Geometry check sheet. Reference: the model listing, model coordinates, mm. Coordinates: 2 decimals unless noted, no trailing zeros. Order: outer loops, then holes, each group sorted by start corner. A loop starts at its lowest first (then second) coordinate and runs counter-clockwise, first axis right, second up. Notation, with made-up numbers: (87, -5) - (95, -5) arc R31 ccw to (95, 30) - close; hole circle Ø7 at (2, 65.5). An arc over 180 degrees is marked (long way). Put each result on its own line as item: value.
from build123d import *

# Parameters (mm, degrees)
SKETCH2_R                = 4
BOSS_EXTRUDE1_DEPTH      = 100
BOSS_EXTRUDE1_2_DEPTH    = 100
BOSS_EXTRUDE3_DEPTH      = 50
BOSS_EXTRUDE3_DEPTH_BACK = 175
BOSS_EXTRUDE4_START      = -15
SKETCH5_R                = 45.011707972
BOSS_EXTRUDE4_DEPTH      = 15
SKETCH8_R                = 30.011707972
CUT_EXTRUDE1_DEPTH       = 210


with BuildPart() as part:
    # Sketch2 → Boss-Extrude1 (new body)
    with BuildSketch(Plane(origin=(0, 0, 0), x_dir=(-1, 0, 0), z_dir=(0, 0.499999999999998, -0.8660254037844398))):
        with Locations(Location((-17.5, 0, 0), (0, 0, 90))):
            Circle(SKETCH2_R)
    boss_extrude1 = extrude(amount=BOSS_EXTRUDE1_DEPTH)



with BuildPart() as body_2:
    # Sketch2 → Boss-Extrude1 2 (new body)
    with BuildSketch(Plane(origin=(0, 0, 0), x_dir=(-1, 0, 0), z_dir=(0, 0.499999999999998, -0.8660254037844398))):
        with Locations(Location((17.5, 0, 0), (0, 0, 90))):
            Circle(SKETCH2_R)
    boss_extrude1_2 = extrude(amount=BOSS_EXTRUDE1_2_DEPTH)


with BuildPart() as part_1:
    add(part.part)

    add(body_2.part)  # Boss-Extrude3 merges body 2
    # Sketch4 → Boss-Extrude3 (add, two sides: drawn at the far end of the back side and taken through both)
    with BuildSketch(Plane(origin=(0, 0, 0), x_dir=(0, 0, 1), z_dir=(-0.9961946980917461, 0.08715574274765156, 0)).offset(-BOSS_EXTRUDE3_DEPTH_BACK)):
        with BuildLine():
            Line((80.028265546, 0), (65.028265546, 0))
            ThreePointArc((65.028265546, 0), (23.531574155, -27.727202731), (13.795075351, 21.221482222))
            Line((13.795075351, 21.221482222), (3.188473633, 31.82808394))
            ThreePointArc((3.188473633, 31.82808394), (17.79132267, -41.585395719), (80.028265546, 0))
        make_face()
    extrude(amount=BOSS_EXTRUDE3_DEPTH + BOSS_EXTRUDE3_DEPTH_BACK)

    # Sketch5 → Boss-Extrude4 (add)
    with BuildSketch(Plane(origin=(-49.809734905, 4.357787137, 0), x_dir=(0, 0, 1), z_dir=(-0.9961946980917462, 0.08715574274765156, 0)).offset(BOSS_EXTRUDE4_START)):
        with Locations(Location((35.016557573, 0, 0), (0, 0, 135))):
            Circle(SKETCH5_R)
    extrude(amount=BOSS_EXTRUDE4_DEPTH)

    # Mirror2: Boss-Extrude1, Boss-Extrude1 2 across plane
    add(boss_extrude1.mirror(Plane(origin=(0, 0, 35.016557573), x_dir=(1, 0, 0), z_dir=(0, 0, -1))))
    add(boss_extrude1_2.mirror(Plane(origin=(0, 0, 35.016557573), x_dir=(1, 0, 0), z_dir=(0, 0, -1))))

    # Sketch8 → Cut-Extrude1 (cut)
    with BuildSketch(Plane(origin=(174.334072166, -15.252254981, 0), x_dir=(0, 0, -1), z_dir=(0.9961946980917462, -0.08715574274765156, 0))):
        with Locations((-35.016557573, 0)):
            Circle(SKETCH8_R)
        with BuildLine():
            Line((-80.028265546, 0), (-208.366954173, 0))
            ThreePointArc((-208.366954173, 0), (87.560683384, -122.577240957), (-35.016557573, 173.3503966))
            Line((-35.016557573, 173.3503966), (-35.016557573, 45.011707972))
            ThreePointArc((-35.016557573, 45.011707972), (-3.188473633, -31.82808394), (-80.028265546, 0))
        make_face()
    extrude(amount=-CUT_EXTRUDE1_DEPTH, mode=Mode.SUBTRACT)


solid = part_1.part
Q1. Section check C-C on z = 47. Record the boundary of the cut face in (x, y).
Answer block:
outline: (-53.59, -38.86) - (170.55, -58.47) - (171.94, -42.66) - (-37.26, -24.36) - (-31.09, 46.27) - (-46.03, 47.58) - close
Q2. Draft check along Z on faces 1 (the cylindrical face through (68.755, -34.155, 24.298)), 2 (the flat face through (-17.444, 49.952, 156.664)), 3 (the flat face through (-49.755, 4.986, 34.386)), 4 (the flat face through (17.556, 0.781, 69.582)). Enter one of: pulls with the +Z half, pulls with the -Z half, needs draft (parallel to the pull), parting line crosses it, or undercut.
Answer block:
face 1: undercut
face 2: pulls with the +Z half
face 3: needs draft
face 4: undercut
Q3. Thickness scan on L1, parallel to Z at x = 67.5, y = -7; L2, parallel to Z at x = -36.5, y = -24; L3, parallel to X at y = -13.5, z = 20.5. Record the ranges inside material, lowest first. Write a range as [from, to].
Answer block:
L1: z = [-9.98, 5.02], [65.01, 80.02]
L2: z = [-0.93, 22.1], [47.93, 70.96]
L3: x = [-51.37, -36.31]
Q4. Section check A-A on z = 22.5. Record the boundary of the cut face in (x, y), then the cut area to 3 significant figures.
Answer block:
outline: (-53.58, -38.71) - (170.57, -58.32) - (171.96, -42.43) - (-37.24, -24.12) - (-31.1, 46.12) - (-46.04, 47.43) - close
area: 4,650 mm^2
Q5. Depth check by flat-ended pin: pin 1 Ø4 at (x, y) = (-9, -8.5) entering from +Z; pin 2 Ø4 at (x, y) = (0.5, -21.5) entering from -Z; pin 3 Ø2 at (x, y) = (75, -14) entering from -Z. Enter the tip coordinate at first touch or a pass-through.
Answer block:
pin 1: stops at z = 79.44
pin 2: stops at z = -5.61
pin 3: stops at z = -9.54
Q6. Section check B-B on y = 27.5. State how many separate pieces and enclosed holes the cut face has, then the cut area to 3 significant figures.
Answer block:
separate pieces: 3
enclosed holes: 0
area: 1,920 mm^2
